from build123d import *

# Parameters (mm, degrees)
SALIENTE_EXTRUIR1_DEPTH = 40
CROQUIS3_R              = 2.5
CORTAR_EXTRUIR1_DEPTH   = 94
CROQUIS5_W              = 40
CROQUIS5_H              = 10
CORTAR_EXTRUIR2_DEPTH   = 40
CROQUIS6_W              = 42
CROQUIS6_H              = 19
CORTAR_EXTRUIR3_DEPTH   = 10
CROQUIS7_R              = 2
CORTAR_EXTRUIR4_DEPTH   = 10


with BuildPart() as part:
    # Croquis2 → Saliente-Extruir1 (new body)
    with BuildSketch(Plane.XY):
        Polygon((-31.145916957, -11.001243781), (-31.145916957, 23.998756219), (53.854083043, 23.998756219), (53.854083043, -11.001243781), (57.854083043, -11.001243781), (57.854083043, 27.998756219), (-35.145916957, 27.998756219), (-35.145916957, -11.001243781), align=None)
    extrude(amount=SALIENTE_EXTRUIR1_DEPTH)

    # Croquis3 → Cortar-Extruir1 (cut, through all)
    with BuildSketch(Plane.ZY.offset(35.145916957)):
        with Locations((20, 7.998756219)):
            Circle(CROQUIS3_R)
    extrude(amount=-CORTAR_EXTRUIR1_DEPTH, mode=Mode.SUBTRACT)

    # Croquis5 → Cortar-Extruir2 (cut)
    with BuildSketch(Plane.ZY.offset(35.145916957)):
        with Locations((20, -6.001243781)):
            Rectangle(CROQUIS5_W, CROQUIS5_H)
    extrude(amount=-CORTAR_EXTRUIR2_DEPTH, mode=Mode.SUBTRACT)

    # Croquis6 → Cortar-Extruir3 (cut)
    with BuildSketch(Plane(origin=(0, 27.998756219, 0), x_dir=(1, 0, 0), z_dir=(0, 1, 0))):
        with Locations((11.354083043, -20)):
            Rectangle(CROQUIS6_W, CROQUIS6_H)
    extrude(amount=-CORTAR_EXTRUIR3_DEPTH, mode=Mode.SUBTRACT)

    # Croquis7 → Cortar-Extruir4 (cut)
    with BuildSketch(Plane(origin=(0, 27.998756219, 0), x_dir=(1, 0, 0), z_dir=(0, 1, 0))):
        with Locations((-13.645916957, -15)):
            Circle(CROQUIS7_R)
        with Locations((-13.645916957, -25)):
            Circle(CROQUIS7_R)
        with Locations((36.354083043, -15)):
            Circle(CROQUIS7_R)
        with Locations((36.354083043, -25)):
            Circle(CROQUIS7_R)
    extrude(amount=-CORTAR_EXTRUIR4_DEPTH, mode=Mode.SUBTRACT)


solid = part.part
Read the model definition and answer for the solid it produces. Units are mm, in the model's axes. A direction names the side the tool comes from. Give positions to 0.01 mm unless a question says otherwise; leave off trailing zeros. Write each loop counter-clockwise with the first axis right and the second up, starting at its lowest first coordinate (ties: lowest second). Pieces come first, ordered by that corner, then holes. Notation, with made-up numbers: (75, 81.25) - (115, 81.25) arc R21 cw to (115, 114.25) - close; hole circle Ø6 at (87, 16). An arc over 180 degrees is marked (long way). Return JSON: item names as keys, results as strings.
Q1. A cutting plane is placed at A-A, the plane y = 22.5. Determine the outline of the cut face in (x, z).
Reply:
{"outline": "(-35.15, 0) - (-31.15, 0) - (-31.15, 40) - (-35.15, 40) - close; (53.85, 0) - (57.85, 0) - (57.85, 40) - (53.85, 40) - close"}
Q2. For a pull along X with two mould halves and no side action, classify faces 4 (the face through (55.826, 8.109, 17.502)), 5 (the face through (-35.146, 14, 20)), 6 (the face through (-13.906, 26.027, 13.017)) as released by +X, released by -X, zero draft, split by the parting line, or undercut.
Reply:
{"face 4": "zero draft", "face 5": "released by -X", "face 6": "undercut"}
Q3. A cutting plane is placed at D-D, the plane z = 34. Determine the outline of the cut face in (x, y).
Reply:
{"outline": "(-35.15, -1) - (-31.15, -1) - (-31.15, 24) - (53.85, 24) - (53.85, -11) - (57.85, -11) - (57.85, 28) - (-35.15, 28) - close"}
Q4. Consider line 1 along X through (y, z) = (25, 15); line 2 along Y through (x, z) = (55, 20); line 3 along X through (y, z) = (21, 29). Determine where each line is inside the solid, lowest interval first. Write a range as [from, to].
Reply:
{"line 1": "[-35.15, -15.65], [-11.65, -9.65], [32.35, 34.35], [38.35, 57.85]", "line 2": "[-11, 5.5], [10.5, 28]", "line 3": "[-35.15, -31.15], [53.85, 57.85]"}
Q5. A cutting plane is placed at C-C, the plane x = 18. Determine the outline of the cut face in (y, z), and give its area (3 significant figures).
Reply:
{"outline": "(24, 0) - (28, 0) - (28, 10.5) - (24, 10.5) - close; (24, 29.5) - (28, 29.5) - (28, 40) - (24, 40) - close", "area": "84.0 mm²"}
Q6. Given P1, Ø2.5, axis at x = -13.65, z = 15, coming from the -Y side; P2, Ø1.2, axis at x = -32.5, z = 17.5, coming from the -Y side; P3, Ø20, axis at x = 28.5, z = 20.5, coming from the -Y side; P4, Ø5, axis at x = 36.35, z = 25, coming from the +Y side, each flat-ended and moving along its own axis, determine where each tip first touches the part or whether it passes through.
Reply:
{"P1": "through", "P2": "y = -1", "P3": "y = 24", "P4": "y = 28"}
Q7. For faces 1 (the face through (-31.146, 11, 20)), 2 (the face through (-9.646, 26, 20)), 3 (the face through (14.6, 24.5, 40)), determine the directions among +Z, -Z, +X, -X, +Y, -Y from which every point of the face is accessible in a straight line to the end or side of a thin tool.
Reply:
{"face 1": "+Z, -Z, -Y", "face 2": "+Y, -Y", "face 3": "+Z, +X, -X, +Y, -Y"}
Q8. A cutting plane is placed at B-B, the plane z = 20. Determine the outline of the cut face in (x, y), and give its area (3 significant figures).
Reply:
{"outline": "(-35.15, -1) - (-31.15, -1) - (-31.15, 5.5) - (-35.15, 5.5) - close; (-35.15, 10.5) - (-31.15, 10.5) - (-31.15, 24) - (-9.65, 24) - (-9.65, 28) - (-35.15, 28) - close; (32.35, 24) - (53.85, 24) - (53.85, 10.5) - (57.85, 10.5) - (57.85, 28) - (32.35, 28) - close; (53.85, -11) - (57.85, -11) - (57.85, 5.5) - (53.85, 5.5) - close", "area": "404 mm²"}
